For this review, take the finished solid that the model builds, in its own axes (mm). Face numbers are marked on the shaded views. A direction names the side the tool comes from. Give positions to 0.01 mm unless a question says otherwise; leave off trailing zeros. Loops run counter-clockwise (first coordinate to the right, second up) from the corner with the lowest first, then second, coordinate; pieces in that order, holes last. Notation, with made-up numbers: (51.5, 45) - (85.5, 45) arc R20 cw to (85.5, 75) - close; hole circle Ø11 at (2.25, -28). An arc over 180 degrees is marked (long way). Use CSV: the item, a comma, the result in double quotes. Start each with the question number.
1. Take a section at D-D on z = 3. Give the boundary of the cut face in (x, y).
2. Mouldability with a two-part tool opening along Y and no side actions: class the marked faces 1, 2 and 3 as pulls with the +Y half, pulls with the -Y half, needs draft (parallel to the pull), parting line crosses it, or undercut.
3. Take a section at B-B on x = 0. Give the boundary of the cut face in (y, z).
4. Take a section at A-A on z = 0. Give the boundary of the cut face in (x, y).
5. For the marked faces 4 and 5, list the 3-axis set-ups (+Z, -Z, +X, -X, +Y, -Y) from which the entire face can be reached by the end or side of a thin tool; tool diameter is ignored.
6. For pin 1 (3 mm diameter, centred on y = 2, z = 2, fed in from +X); pin 2 (1.5 mm diameter, centred on x = -1.5, y = 12, fed in from -Z), all flat-tipped, find the tip position at first contact; note any pin that passes through.
7. Take a section at C-C on y = 4.75. Give the boundary of the cut face in (x, z), plus the area to 3 significant figures.
8. Wall thickness on line 1 (Z direction, x = 0, y = 11.75); line 2 (Y direction, x = 3, z = 0): over which ranges is each line inside the solid? List them lowest first.
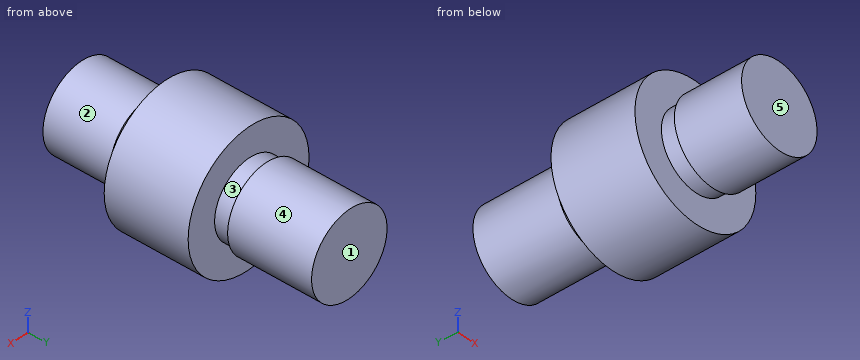
Autodesk Inventor part; units mm, degrees
ref_plane "YZ Plane" through (0, 0, 0) normal (1, 0, 0) x (0, 1, 0)
ref_plane "XZ Plane" through (0, 0, 0) normal (0, 1, 0) x (-1, 0, 0)
ref_plane "XY Plane" through (0, 0, 0) normal (0, 0, 1) x (1, 0, 0)
sketch "Sketch1" plane through (0, 0, 0) normal (0, 1, 0) x (-1, 0, 0)
  circle A0 centre (0, 0) radius 2.5
  dimension "d0" = 5
extrude "Extrusion1" add sketch "Sketch1" along normal blind 4
sketch "Sketch2" plane through (0, 4, 0) normal (0, 1, 0) x (1, 0, 0)
  circle A0 centre (0, 0) radius 2.25
  dimension "d3" = 4.5
extrude "Extrusion2" add sketch "Sketch2" along normal blind 1
sketch "Sketch3" plane through (0, 5, 0) normal (0, 1, 0) x (1, 0, 0)
  circle A0 centre (0, 0) radius 4
  dimension "d6" = 8
extrude "Extrusion3" add sketch "Sketch3" along normal blind 5
sketch "Sketch4" plane through (0, 10, 0) normal (0, 1, 0) x (1, 0, 0)
  circle A0 centre (0, 0) radius 2.25
  dimension "d9" = 4.5
extrude "Extrusion4" add sketch "Sketch4" along normal blind 1
sketch "Sketch5" plane through (0, 11, 0) normal (0, 1, 0) x (1, 0, 0)
  circle A0 centre (0, 0) radius 2.5
  dimension "d18" = 5
extrude "Extrusion5" add sketch "Sketch5" along normal blind 5
thread "Thread1"
thread "Thread2"
properties part number "Cylinder Piping connector" material "Brass, Soft Yellow"
Check result:
1,outline,"(-2.65, 5) - (2.65, 5) - (2.65, 10) - (-2.65, 10) - close"
2,face 1,"pulls with the +Y half"
2,face 2,"needs draft"
2,face 3,"undercut"
3,outline,"(0, -2.5) - (4, -2.5) - (4, -2.25) - (5, -2.25) - (5, -4) - (10, -4) - (10, -2.25) - (11, -2.25) - (11, -2.5) - (16, -2.5) - (16, 2.5) - (11, 2.5) - (11, 2.25) - (10, 2.25) - (10, 4) - (5, 4) - (5, 2.25) - (4, 2.25) - (4, 2.5) - (0, 2.5) - close"
4,outline,"(-4, 5) - (-2.25, 5) - (-2.25, 4) - (-2.5, 4) - (-2.5, 0) - (2.5, 0) - (2.5, 4) - (2.25, 4) - (2.25, 5) - (4, 5) - (4, 10) - (2.25, 10) - (2.25, 11) - (2.5, 11) - (2.5, 16) - (-2.5, 16) - (-2.5, 11) - (-2.25, 11) - (-2.25, 10) - (-4, 10) - close"
5,face 4,"+Y"
5,face 5,"+Z, -Z, +X, -X, -Y"
6,pin 1,"stops at x = 2.45"
6,pin 2,"stops at z = -2.38"
7,outline,"circle Ø4.5 at (0, 0)"
7,area,"15.9 mm²"
8,line 1,"z = -2.5 to 2.5"
8,line 2,"y = 5 to 10"
